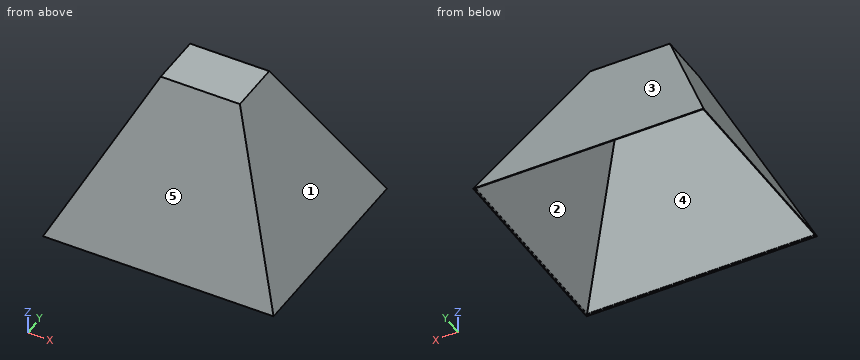
from build123d import *

# Parameters (mm, degrees)
SKETCH1_W           = 350
SKETCH1_H           = 310
BOSS_EXTRUDE1_DEPTH = 235.7
BOSS_EXTRUDE1_TAPER = 26
SHELL1_T            = -1
SKETCH3_W           = 346
SKETCH3_H           = 306
CUT_EXTRUDE1_DEPTH  = 2


with BuildPart() as part:
    # Sketch1 → Boss-Extrude1 (new body)
    with BuildSketch(Plane.XY):
        Rectangle(SKETCH1_W, SKETCH1_H)
    extrude(amount=BOSS_EXTRUDE1_DEPTH, taper=BOSS_EXTRUDE1_TAPER)

    # Shell1
    shell1_openings = [part.faces().sort_by_distance(p)[0] for p in [
        (0, 0, 0),
    ]]
    offset(amount=SHELL1_T, openings=shell1_openings, kind=Kind.INTERSECTION)

    # Sketch3 → Cut-Extrude1 (cut)
    with BuildSketch(Plane(origin=(0, 0, 0), x_dir=(-1, 0, 0), z_dir=(0, 0, -1))):
        Rectangle(SKETCH3_W, SKETCH3_H)
    extrude(amount=-CUT_EXTRUDE1_DEPTH, mode=Mode.SUBTRACT)


solid = part.part
Check sheet for the modelled part. Datum: model origin and axes. Units: mm. Face numbers are marked on the shaded views. A direction names the side the tool comes from. Round coordinates to 2 decimals unless told otherwise and drop trailing zeros. Loops run counter-clockwise (first coordinate to the right, second up) from the corner with the lowest first, then second, coordinate; pieces in that order, holes last. Notation, with made-up numbers: (-24.75, -28.75) -> (-5.75, -28.75) arc R33 ccw to (-5.75, 4.25) -> close; hole circle Ø7 at (89.5, 20). An arc over 180 degrees is marked (long way). Put each result on its own line as item: value. Start each with the question number.
1. Section check B-B (x = -13). Enter the section's corners in (y, z).
2. Scan lines: probe 1 along Y at (x, z) = (6, 172.5); probe 2 along Y at (x, z) = (100, 42); probe 3 along X at (y, z) = (66, 144.5). Record each from-to range of solid material in increasing order.
3. Section check A-A (z = 105.5). Enter the section's corners in (x, y).
4. Draft check along Y on the marked faces 3, 4 and 5. Enter one of: +Y half, -Y half, draft (parallel to the pull), parting line (faces both ways), or undercut.
5. Gauge pin test, flat ends, axial feed: pin 1 (1 mm diameter, centred on x = -36, y = 78.5, fed in from -Z); pin 2 (1 mm diameter, centred on x = 33.5, z = 186, fed in from -Y); pin 3 (1 mm diameter, centred on x = 39.5, z = 62, fed in from +Y). Record the tip position at first contact, or that the pin passes through.
6. Access from +Z, -Z, +X, -X, +Y, -Y to the whole of each face (thin tool, end or side, straight path). Record for the marked faces 1 and 2.
7. Section check D-D (z = 67). Enter the section's corners in (x, y).
8. Section check C-C (y = 55). Enter the section's corners in (x, z), plus the area to 3 significant figures.
Findings:
1. outline: (-155, 0) -> (-153.89, 0) -> (-153, 1.82) -> (-153, 2) -> (-152.91, 2) -> (-39.42, 234.7) -> (39.42, 234.7) -> (152.91, 2) -> (153, 2) -> (153, 1.82) -> (153.89, 0) -> (155, 0) -> (40.04, 235.7) -> (-40.04, 235.7) -> close
2. probe 1: y = -70.87 to -69.75, 69.75 to 70.87
2. probe 2: y = -134.52 to -133.4, 133.4 to 134.52
2. probe 3: x = -104.52 to -103.41, 103.41 to 104.52
3. outline: (-123.54, -103.54) -> (123.54, -103.54) -> (123.54, 103.54) -> (-123.54, 103.54) -> close; hole (-122.43, -102.43) -> (122.43, -102.43) -> (122.43, 102.43) -> (-122.43, 102.43) -> close
4. face 3: +Y half
4. face 4: undercut
4. face 5: -Y half
5. pin 1: stops at z = 153.54
5. pin 2: stops at y = -64.53
5. pin 3: stops at y = 125
6. face 1: +Z, +X, +Y, -Y
6. face 2: -Z
7. outline: (-142.32, -122.32) -> (142.32, -122.32) -> (142.32, 122.32) -> (-142.32, 122.32) -> close; hole (-141.21, -121.21) -> (141.21, -121.21) -> (141.21, 121.21) -> (-141.21, 121.21) -> close
8. outline: (-175, 0) -> (-173.89, 0) -> (-173, 1.82) -> (-173, 2) -> (-172.91, 2) -> (-75, 202.75) -> (75, 202.75) -> (172.91, 2) -> (173, 2) -> (173, 1.82) -> (173.89, 0) -> (175, 0) -> (75, 205.03) -> (-75, 205.03) -> close
8. area: 796 mm^2
